Geometry check sheet. Reference: the model listing, model coordinates, mm. Face numbers are marked on the shaded views. Round coordinates to 2 decimals unless told otherwise and drop trailing zeros. Write each loop counter-clockwise with the first axis right and the second up, starting at its lowest first coordinate (ties: lowest second). Pieces come first, ordered by that corner, then holes. Notation, with made-up numbers: M 83.5,9.5 L 106.5,9.5 A20 cw 106.5,30.5 Z; hole C 26,-10 d6. An arc over 180 degrees is marked long. Use a Markdown table: item, result.
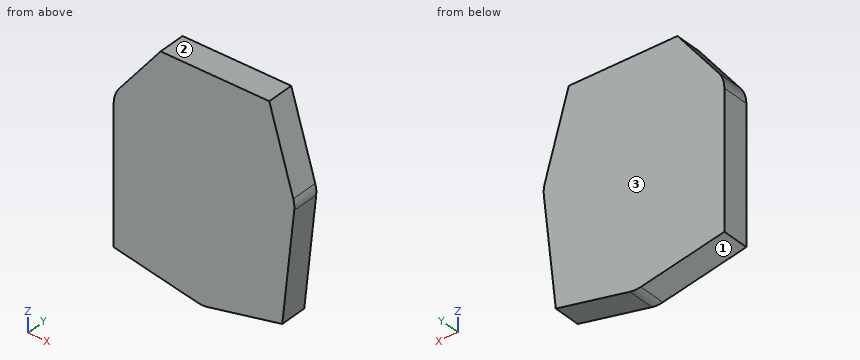
```python
from build123d import *

# Parameters (mm, degrees)
EXTRUDE_1_DEPTH = 15
FILLET_1_R      = 15
FILLET_2_R      = 15
FILLET_3_R      = 15


with BuildPart() as part:
    # Эскиз1 → Бобышка-Вытянуть1 (new body)
    with BuildSketch(Plane(origin=(0, 0, 0), x_dir=(1, 0, 0), z_dir=(0, 1, 0))):
        Polygon((0, 0), (-25.909847732, 33.174508492), (-25.909847732, 113.174508492), (23.200748024, 122.563298857), (67.167075345, 112.973613675), (74.090152268, 47.973613675), (60, 0), align=None)
    extrude(amount=EXTRUDE_1_DEPTH)

    # Скругление1
    fillet_1_edges = [part.edges().sort_by_distance(p)[0] for p in [
        (-25.909847732, 7.5, -33.174508492),
    ]]
    fillet(fillet_1_edges, radius=FILLET_1_R)

    # Скругление2
    fillet_2_edges = [part.edges().sort_by_distance(p)[0] for p in [
        (74.090152268, 7.5, -47.973613675),
    ]]
    fillet(fillet_2_edges, radius=FILLET_2_R)

    # Скругление3
    fillet_3_edges = [part.edges().sort_by_distance(p)[0] for p in [
        (23.200748024, 7.5, -122.563298857),
    ]]
    fillet(fillet_3_edges, radius=FILLET_3_R)


solid = part.part
```
Item 1: Cross-section at C-C, the plane x = 47. Record the cut outline in (y, z).
Outcome:
| item | result |
|---|---|
| outline | M 0,-117.37 L 15,-117.37 L 15,0 L 0,0 Z |
Item 2: Go/stop test with flat-tipped pins: pin 1 (1.5 mm diameter, centred on x = 4.5, y = 4.5, fed in from -Z); pin 2 (8 mm diameter, centred on x = 13, y = 10, fed in from -Z); pin 3 (2 mm diameter, centred on x = 28, y = 4, fed in from -Z). Record where each tip stops, or that it passes through.
Outcome:
| item | result |
|---|---|
| pin 1 | stops at z = -119.13 |
| pin 2 | stops at z = -121.38 |
| pin 3 | stops at z = -121.73 |
Item 3: Cross-section at B-B, the plane z = -84. Record the cut outline in (x, y), and give its area (3 significant figures).
Outcome:
| item | result |
|---|---|
| outline | M -25.91,0 L 70.25,0 L 70.25,15 L -25.91,15 Z |
| area | 1,440 mm2 |
Item 4: Cross-section at A-A, the plane y = 9. Record the cut outline in (x, z), and give its area (3 significant figures).
Outcome:
| item | result |
|---|---|
| outline | M -25.91,-113.17 L 20.19,-121.99 A15 ccw 26.2,-121.91 L 67.17,-112.97 L 73.77,-50.93 A15 ccw 73.25,-45.12 L 60,0 L 0,0 L -22.73,-29.11 A15 ccw -25.91,-38.34 Z |
| area | 10,800 mm2 |
Item 5: Mould release check, pull along Z, two halves, no side actions. Record for the marked faces 1, 2 and 3: +Z half, -Z half, draft (parallel to the pull), parting line (faces both ways), or undercut.
Outcome:
| item | result |
|---|---|
| face 1 | -Z half |
| face 2 | +Z half |
| face 3 | draft |
Item 6: Material ranges on line 1 along Z through (x, y) = (23.5, 2.5); line 2 along X through (y, z) = (11, -39); line 3 along Z through (x, y) = (43, 5.25), recorded low to high. Write a range as from..to.
Outcome:
| item | result |
|---|---|
| line 1 | z = -122.25..0 |
| line 2 | x = -25.91..71.45 |
| line 3 | z = -118.24..0 |
